from build123d import *

# Parameters (mm, degrees)
PAD_DEPTH         = 20
PAD001_DEPTH      = 3
PAD001_DEPTH_BACK = 6


with BuildPart() as part:
    # AdditivePipe: sweep along a path in Sketch
    with BuildLine(Plane.XY) as additivepipe_path:
        Line((0, 0), (0, 47))
    # Sketch001 → AdditivePipe (sweep)
    with BuildSketch(Plane.XZ):
        Polygon((-20, 6), (-20, -6), (-16, -6), (-9, -6), (9, -6), (16, -6), (20, -6), (20, 6), (16, 6), (16, 3), (9, 3), (-9, 3), (-16, 3), (-16, 6), align=None)
    sweep(path=additivepipe_path.line)

    # Sketch002 → Pad (new body, symmetric)
    with BuildSketch(Plane.YZ):
        Polygon((47, 6), (47, 17), (34, 31), (22, 31), (22, 17), (29, 17), (29, 3), (47, 3), align=None)
    extrude(amount=PAD_DEPTH, both=True)

    # Sketch003 → Pad001 (join, two sides)
    with BuildSketch(Plane.XY) as pad001_sk:
        with BuildLine():
            Line((-3, 0), (3, 0))
            Line((3, 0), (3, -8))
            ThreePointArc((-3, -8), (0, -17), (3, -8))
            Line((-3, 0), (-3, -8))
        make_face()
    extrude(amount=PAD001_DEPTH)
    extrude(pad001_sk.sketch, amount=-PAD001_DEPTH_BACK)


solid = part.part
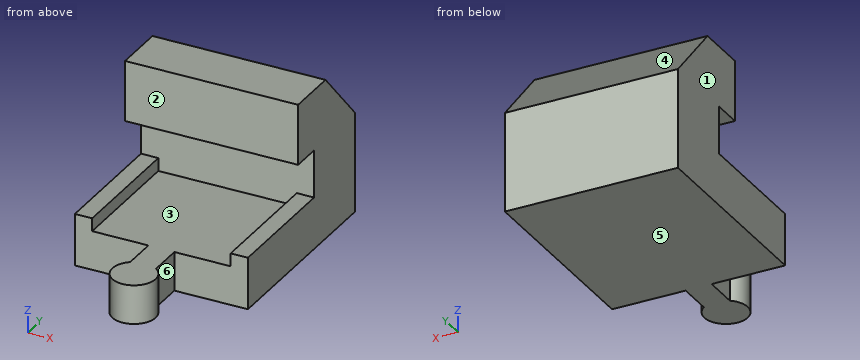
Check sheet for the modelled part. Datum: model origin and axes. Units: mm. Face numbers are marked on the shaded views. A direction names the side the tool comes from. Give positions to 0.01 mm unless a question says otherwise; leave off trailing zeros. Order: outer loops, then holes, each group sorted by start corner. A loop starts at its lowest first (then second) coordinate and runs counter-clockwise, first axis right, second up. Notation, with made-up numbers: M 85,25 L 99,25 A18 cw 99,59 Z; hole C 74.5,74.5 d2. An arc over 180 degrees is marked long. Answer as CSV lines item,"result". Start each with the question number.
Item 1: Mould release check, pull along Y, two halves, no side actions. Record for the marked faces 4, 5 and 6: +Y half, -Y half, draft (parallel to the pull), parting line (faces both ways), or undercut.
Item 2: Cross-section at A-A on x = -10.5. Enter the section's corners in (y, z).
Item 3: Tool access check on the marked faces 1, 2 and 3. Record the directions out of +Z, -Z, +X, -X, +Y, -Y that give a thin tool (end or side, any length) a straight path to the whole face; none if there is none.
Item 4: Thickness scan on line 1 (X direction, y = 6.5, z = 4.5); line 2 (Z direction, x = 12, y = 7.5); line 3 (Y direction, x = 2.5, z = 15). Record the ranges inside material, lowest first. Write a range as [from, to].
Item 5: Cross-section at D-D on y = -12. Enter the section's corners in (x, z), plus the area to 3 significant figures.
Item 6: Cross-section at C-C on x = 0. Enter the section's corners in (y, z).
Item 7: Cross-section at B-B on y = 16. Enter the section's corners in (x, z), plus the area to 3 significant figures.
Item 8: Gauge pin test, flat ends, axial feed: P1, Ø4, axis at x = -4, z = 22, coming from the -Y side; P2, Ø8, axis at x = 4.5, y = 17.5, coming from the +Z side; P3, Ø4.5, axis at x = 17.5, y = 10, coming from the +Z side. Record the tip position at first contact, or that the pin passes through.
Established:
1,face 4,"+Y half"
1,face 5,"draft"
1,face 6,"undercut"
2,outline,"M 0,-6 L 47,-6 L 47,17 L 34,31 L 22,31 L 22,17 L 29,17 L 29,3 L 0,3 Z"
3,face 1,"+Z, -Z, -X, +Y, -Y"
3,face 2,"+Z, +X, -X, -Y"
3,face 3,"-Y"
4,line 1,"x = [-20, -16], [16, 20]"
4,line 2,"z = [-6, 3]"
4,line 3,"y = [29, 47]"
5,outline,"M -5,-6 L 5,-6 L 5,3 L -5,3 Z"
5,area,"90.0 mm^2"
6,outline,"M -17,-6 L 47,-6 L 47,17 L 34,31 L 22,31 L 22,17 L 29,17 L 29,3 L -17,3 Z"
7,outline,"M -20,-6 L 20,-6 L 20,6 L 16,6 L 16,3 L -16,3 L -16,6 L -20,6 Z"
7,area,"384 mm^2"
8,P1,"stops at y = 22"
8,P2,"stops at z = 3"
8,P3,"stops at z = 6"
